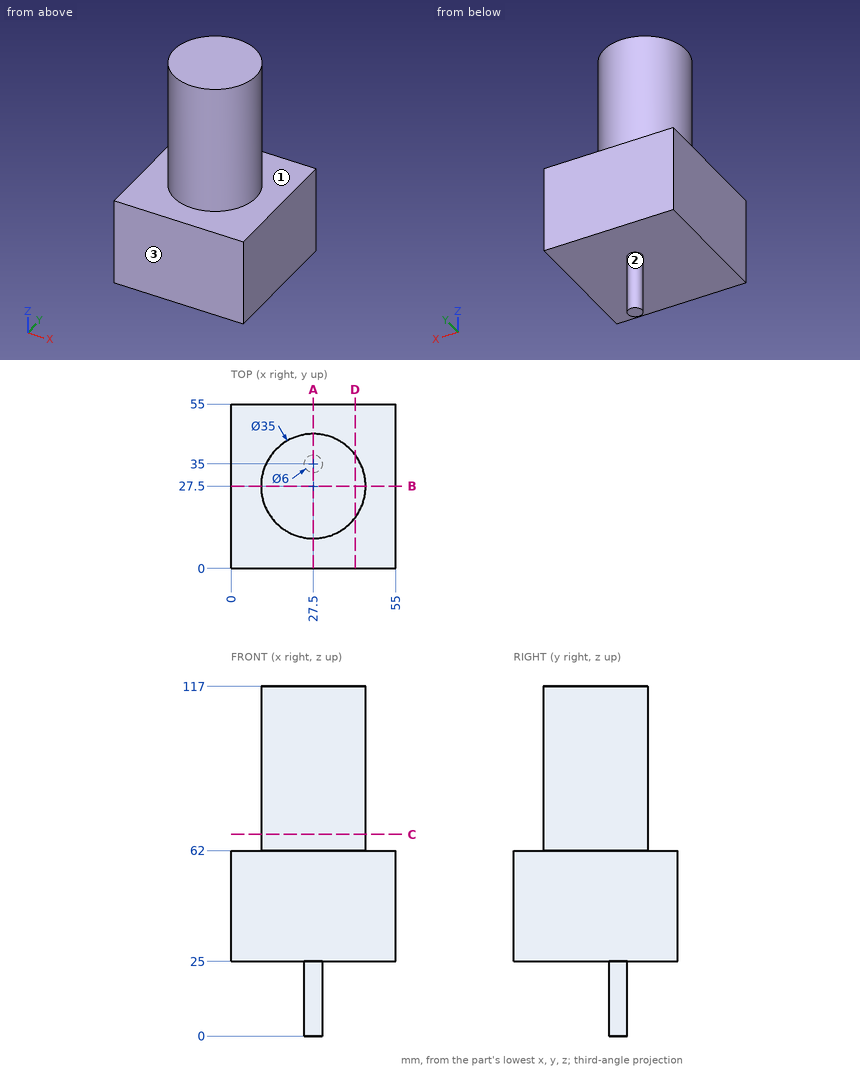
Study the drawing (mm; zero at the part's minimum x, y, z) and answer. A direction names the side the tool comes from. Give positions to 0.01 mm unless a question says otherwise; leave off trailing zeros. Write each loop counter-clockwise with the first axis right and the second up, starting at its lowest first coordinate (ties: lowest second). Pieces come first, ordered by that corner, then holes. Notation, with made-up numbers: (35.25, 79.5) - (50.25, 79.5) arc R22 ccw to (50.25, 101.5) - close; hole circle Ø7 at (-10.5, 70.25). An arc over 180 degrees is marked (long way). Use CSV: the item, a comma, the result in double quotes. Start each with the question number.
(1) Find section A-A (x = 27.5). Give the vertices of the cut face in (y, z), plus the area to 3 significant figures.
(2) Find section D-D (x = 41.5). Give the vertices of the cut face in (y, z), plus the area to 3 significant figures.
(3) Find section B-B (y = 27.5). Give the vertices of the cut face in (x, z).
(4) Given P1, Ø5, axis at x = 13, y = 6, coming from the -Z side; P2, Ø1, axis at x = 46.5, z = 41.5, coming from the -Y side; P3, Ø3, axis at x = 47.5, y = 23.5, coming from the +Z side; P4, Ø2, axis at y = 17, z = 87.5, coming from the -X side, each flat-ended and moving along its own axis, determine where each tip first touches the part or whether it passes through.
(5) Find section C-C (z = 67.5). Give the vertices of the cut face in (x, y).
(6) Consider line 1 along Z through (x, y) = (35.5, 8.5); line 2 along Z through (x, y) = (38, 36.5); line 3 along X through (y, z) = (15, 74). Determine where each line is inside the solid, lowest interval first.
(7) For the marked faces 1, 2 and 3, determine the directions among +Z, -Z, +X, -X, +Y, -Y from which every point of the face is accessible in a straight line to the end or side of a thin tool.
Findings below:
1,outline,"(0, 25) - (32, 25) - (32, 0) - (38, 0) - (38, 25) - (55, 25) - (55, 62) - (45, 62) - (45, 117) - (10, 117) - (10, 62) - (0, 62) - close"
1,area,"4,110 mm2"
2,outline,"(0, 25) - (55, 25) - (55, 62) - (38, 62) - (38, 117) - (17, 117) - (17, 62) - (0, 62) - close"
2,area,"3,190 mm2"
3,outline,"(0, 25) - (55, 25) - (55, 62) - (45, 62) - (45, 117) - (10, 117) - (10, 62) - (0, 62) - close"
4,P1,"z = 25"
4,P2,"y = 0"
4,P3,"z = 62"
4,P4,"x = 12.8"
5,outline,"circle Ø35 at (27.5, 27.5)"
6,line 1,"25 to 62"
6,line 2,"25 to 117"
6,line 3,"15.25 to 39.75"
7,face 1,"+Z"
7,face 2,"-Z"
7,face 3,"+Z, -Z, +X, -X, -Y"
